```python
from build123d import *

# Parameters (mm, degrees)
F0_R     = 2.75
F1_DEPTH = 3


with BuildPart() as f1:
    # F0 (on Front) → F1 (new body)
    with BuildSketch(Plane.XZ):
        Polygon((-17, 0), (0, 0), (0, 7), (3, 7), (3, 17), (0, 17), (0, 24), (3, 24), (3, 34), (0, 34), (0, 41), (-17, 41), (-17, 44), (-27, 44), (-27, 41), (-36, 41), (-36, 37.5), (-34.891142, 37.5), (-34.891142, 35.5), (-36, 35.5), (-36, 29), (-37.782284, 29), (-37.782284, 35.5), (-38.891142, 35.5), (-38.891142, 37.5), (-37.782284, 37.5), (-37.782284, 40.915333), (-47, 41), (-47, 44), (-57, 44), (-57, 41), (-66.217716, 41), (-66.217716, 37.5), (-65.108858, 37.5), (-65.108858, 35.5), (-66.217716, 35.5), (-66.217716, 29), (-68, 29), (-68, 35.5), (-69.108858, 35.5), (-69.108858, 37.5), (-68, 37.5), (-68, 41), (-77, 41), (-77, 44), (-87, 44), (-87, 41), (-104, 41), (-104, 34), (-107, 34), (-107, 24), (-104, 24), (-104, 17), (-107, 17), (-107, 7), (-104, 7), (-104, 0), (-87, 0), (-87, -3), (-77, -3), (-77, 0), (-68, 0), (-68, 6.5), (-69, 6.5), (-69, 8.5), (-68, 8.5), (-68, 12), (-66, 12), (-66, 8.5), (-65, 8.5), (-65, 6.5), (-66, 6.5), (-66, 0), (-57, 0), (-57, -3), (-47, -3), (-47, 0), (-38, 0), (-38, 6.5), (-39, 6.5), (-39, 8.5), (-38, 8.5), (-38, 12), (-36, 12), (-36, 8.5), (-35, 8.5), (-35, 6.5), (-36, 6.5), (-36, 0), (-27, 0), (-27, -3), (-17, -3), align=None)
        with Locations((-13.5, 20.5)):
            Circle(F0_R, mode=Mode.SUBTRACT)
    extrude(amount=F1_DEPTH)


solid = f1.part
```
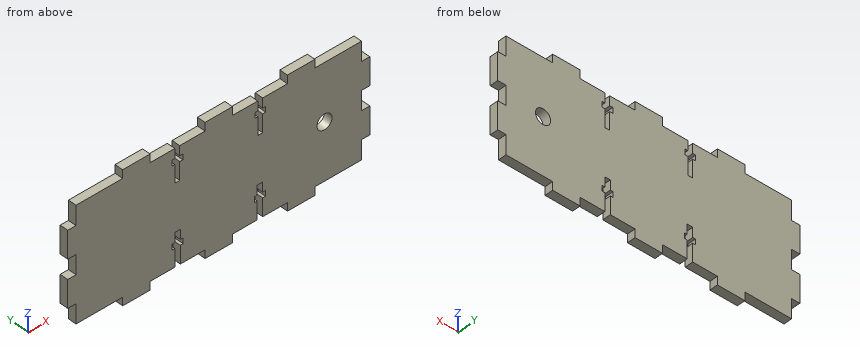
CAD build for the part. Positions are in the model's coordinates, mm. Round coordinates to 2 decimals unless told otherwise and drop trailing zeros. Loops run counter-clockwise (first coordinate to the right, second up) from the corner with the lowest first, then second, coordinate; pieces in that order, holes last. Notation, with made-up numbers: (11.5, 52.25) - (64.5, 52.25) arc R20 ccw to (64.5, 78.25) - close; hole circle Ø10 at (11.25, -8.75). An arc over 180 degrees is marked (long way). Return JSON: item names as keys, results as strings. Group by question number.
Q1. Flat gauge pins, fed straight in: pin 1 Ø1.5 at (x, y) = (-37, -1.5) entering from +Z; pin 2 Ø0.9 at (y, z) = (-2, 2.5) entering from +X. Where does each tip first touch, or does it go through?
Q2. Band-saw the part on A-A on x = -13.5. Give the cut face in (y, z).
Q3. Band-saw the part on C-C on z = 39. Give the cut face in (x, y), plus the area to 3 significant figures.
Q4. Band-saw the part on D-D on x = -46. Give the cut face in (y, z).
Q5. Band-saw the part on B-B on z = 20.5. Give the cut face in (x, y).
Q6. Drill centre lines: line 1 along X through (y, z) = (-1.9, 30.5); line 2 along X through (y, z) = (-0.3, 1); line 3 along Z through (x, y) = (-13.5, -0.7). Where is each one in solid material? Low to high. Write a range as [from, to].
Solutions:
{
 "1": {"pin 1": "stops at z = 29", "pin 2": "stops at x = 0"},
 "2": {"outline": "(-3, 0) - (0, 0) - (0, 17.75) - (-3, 17.75) - close; (-3, 23.25) - (0, 23.25) - (0, 41) - (-3, 41) - close"},
 "3": {"outline": "(-104, -3) - (-68, -3) - (-68, 0) - (-104, 0) - close; (-66.22, -3) - (-37.78, -3) - (-37.78, 0) - (-66.22, 0) - close; (-36, -3) - (0, -3) - (0, 0) - (-36, 0) - close", "area": "301 mm^2"},
 "4": {"outline": "(-3, 0) - (0, 0) - (0, 40.99) - (-3, 40.99) - close"},
 "5": {"outline": "(-104, -3) - (-16.25, -3) - (-16.25, 0) - (-104, 0) - close; (-10.75, -3) - (0, -3) - (0, 0) - (-10.75, 0) - close"},
 "6": {"line 1": "x = [-107, -68], [-66.22, -37.78], [-36, 3]", "line 2": "x = [-104, -68], [-66, -38], [-36, 0]", "line 3": "z = [0, 17.75], [23.25, 41]"}
}
